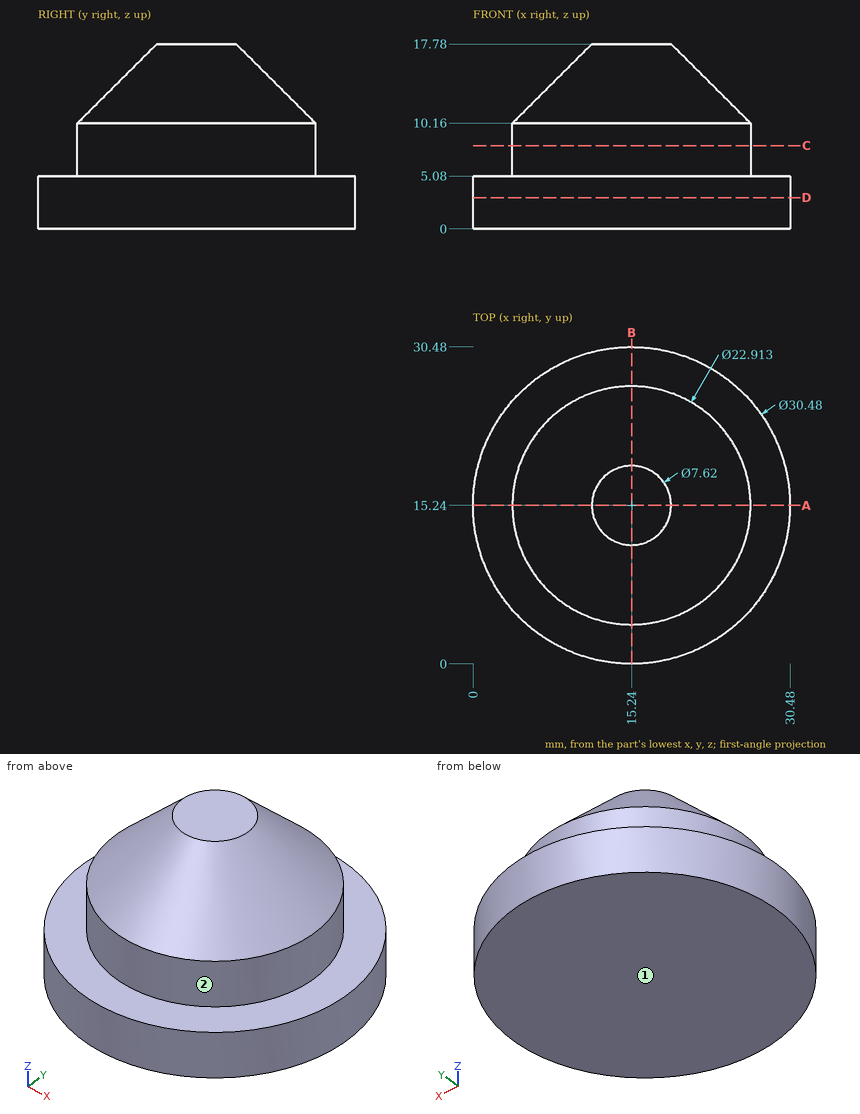
Part print with two shaded views. Sizes in mm from the minimum x, y, z corner. A direction names the side the tool comes from. Coordinates: 2 decimals unless noted, no trailing zeros. Loops run counter-clockwise (first coordinate to the right, second up) from the corner with the lowest first, then second, coordinate; pieces in that order, holes last. Notation, with made-up numbers: (-35.75, 28) -> (8.25, 28) arc R11 cw to (8.25, 46) -> close; hole circle Ø6 at (31.5, 46.25). An arc over 180 degrees is marked (long way). Answer as a JSON object with one key per item and string values.
Q1. 3-axis set-ups, long thin cutter, end or side, ignore diameter. For the marked faces 1 and 2: which of +Z, -Z, +X, -X, +Y, -Y reach the whole face in a straight line?
Report:
{"face 1": "-Z, +X, -X, +Y, -Y", "face 2": "+Z"}
Q2. Flat gauge pins, fed straight in: P1, Ø6, axis at y = 26.5, z = 10, coming from the +X side; P2, Ø2, axis at x = 9, z = 14, coming from the +Y side (1 decimal); P3, Ø3, axis at x = 25, z = 3.5, coming from the -Y side. Where does each tip first touch, or does it go through?
Report:
{"P1": "stops at x = 23.18", "P2": "stops at y = 21.5", "P3": "stops at y = 2.43"}
Q3. Cut at D-D (z = 3). List the corners of the cut face in (x, y), and give its area (3 significant figures).
Report:
{"outline": "circle Ø30.48 at (15.24, 15.24)", "area": "730 mm2"}
Q4. Cut at C-C (z = 8). List the corners of the cut face in (x, y), and give its area (3 significant figures).
Report:
{"outline": "circle Ø22.91 at (15.24, 15.24)", "area": "412 mm2"}
Q5. Cut at A-A (y = 15.24). List the corners of the cut face in (x, z), and give its area (3 significant figures).
Report:
{"outline": "(0, 0) -> (30.48, 0) -> (30.48, 5.08) -> (26.7, 5.08) -> (26.7, 10.16) -> (19.05, 17.78) -> (11.43, 17.78) -> (3.78, 10.16) -> (3.78, 5.08) -> (0, 5.08) -> close", "area": "388 mm2"}
Q6. Probe probe 1 along Z at (x, y) = (3, 20); probe 2 along Y at (x, z) = (21, 6.25); probe 3 along Y at (x, z) = (28.5, 2). List the from-to ranges inside material, lowest first.
Report:
{"probe 1": "z = 0 to 5.08", "probe 2": "y = 5.34 to 25.14", "probe 3": "y = 7.73 to 22.75"}
